from build123d import *

# Parameters (mm, degrees)
F1_DEPTH = 6.8
F3_DEPTH = 25
F5_DEPTH = 2
F7_DEPTH = 2


with BuildPart() as f1:
    # F0 (on Top) → F1 (new body)
    with BuildSketch(Plane.XY):
        with BuildLine():
            ThreePointArc((-46.538709, 10.046789), (-53.609776, 7.117857), (-56.538709, 0.046789))
            Line((-56.538709, 0.046789), (-37.538709, 0.046789))
            Line((-37.538709, 0.046789), (-37.538709, 10.046789))
            Line((-37.538709, 10.046789), (-46.538709, 10.046789))
        make_face()
        with BuildLine():
            Line((-37.538709, 0.046789), (-56.538709, 0.046789))
            ThreePointArc((-56.538709, 0.046789), (-53.609776, -7.024279), (-46.538709, -9.953211))
            Line((-46.538709, -9.953211), (-37.538709, -9.953211))
            Line((-37.538709, -9.953211), (-37.538709, 0.046789))
        make_face()
        with BuildLine():
            Line((-37.538709, 10.046789), (-37.538709, 0.046789))
            Line((-37.538709, 0.046789), (-18.538709, 0.046789))
            ThreePointArc((-18.538709, 0.046789), (-21.467641, 7.117857), (-28.538709, 10.046789))
            Line((-28.538709, 10.046789), (-37.538709, 10.046789))
        make_face()
        with BuildLine():
            Line((-18.538709, 0.046789), (-37.538709, 0.046789))
            Line((-37.538709, 0.046789), (-37.538709, -9.953211))
            Line((-37.538709, -9.953211), (-28.538709, -9.953211))
            ThreePointArc((-28.538709, -9.953211), (-21.467641, -7.024279), (-18.538709, 0.046789))
        make_face()
    extrude(amount=F1_DEPTH)

    # F2 (on face) → F3 (cut)
    with BuildSketch(Plane.XZ.offset(9.953211)):
        with BuildLine():
            Line((-46.538709, 6.8), (-46.538709, 4.885035))
            add(Edge.make_bspline(
                [(-46.538709, 4.885035), (-37.538709, 3.536233), (-28.538709, 4.885035)],
                knots=[4.014167, 4.014167, 4.014167, 5.410611, 5.410611, 5.410611], degree=2, weights=[1, 0.765986, 1]))
            Line((-28.538709, 4.885035), (-28.538709, 6.8))
            Line((-28.538709, 6.8), (-46.538709, 6.8))
        make_face()
        with BuildLine():
            add(Edge.make_bspline(
                [(-28.538709, 4.885035), (-23.538709, 5.634369), (-23.538709, 6.8)],
                knots=[5.410611, 5.410611, 5.410611, 6.283185, 6.283185, 6.283185], degree=2, weights=[1, 0.906327, 1]))
            add(Edge.make_bspline(
                [(-23.538709, 6.8), (-23.538709, 10.724017), (-43.454788, 9.065817), (-63.370868, 7.407617), (-46.538709, 4.885035)],
                knots=[0, 0, 0, 2.007083, 2.007083, 4.014167, 4.014167, 4.014167], degree=2, weights=[1, 0.537319, 1, 0.537319, 1]))
            Line((-46.538709, 4.885035), (-46.538709, 6.8))
            Line((-46.538709, 6.8), (-28.538709, 6.8))
            Line((-28.538709, 6.8), (-28.538709, 4.885035))
        make_face()
    extrude(amount=-F3_DEPTH, mode=Mode.SUBTRACT)

    # F4 (on face) → F5 (cut)
    with BuildSketch(Plane(origin=(0, 0, 0), x_dir=(1, 0, 0), z_dir=(0, 0, -1))):
        with BuildLine():
            Line((-28.538709, 9.353211), (-46.538709, 9.353211))
            ThreePointArc((-46.538709, 9.353211), (-55.938709, -0.046789), (-46.538709, -9.446789))
            Line((-46.538709, -9.446789), (-28.538709, -9.446789))
            ThreePointArc((-28.538709, -9.446789), (-19.138709, -0.046789), (-28.538709, 9.353211))
        make_face()
    extrude(amount=-F5_DEPTH, mode=Mode.SUBTRACT)

    # F6 (on face) → F7 (cut)
    with BuildSketch(Plane(origin=(0, 0, 2), x_dir=(1, 0, 0), z_dir=(0, 0, -1))):
        with BuildLine():
            Line((-28.538709, 3.953211), (-46.538709, 3.953211))
            ThreePointArc((-46.538709, 3.953211), (-50.538709, -0.046789), (-46.538709, -4.046789))
            Line((-46.538709, -4.046789), (-28.538709, -4.046789))
            ThreePointArc((-28.538709, -4.046789), (-24.538709, -0.046789), (-28.538709, 3.953211))
        make_face()
    extrude(amount=-F7_DEPTH, mode=Mode.SUBTRACT)


solid = f1.part
The listing builds one solid part. Answer for the finished solid, in the listing's coordinates (mm). A direction names the side the tool comes from. Give positions to 0.01 mm unless a question says otherwise; leave off trailing zeros. Loops run counter-clockwise (first coordinate to the right, second up) from the corner with the lowest first, then second, coordinate; pieces in that order, holes last.
Item 1: Each of these flat-tipped pins is pushed along its axis until it touches: pin 1 Ø5.5 at (x, y) = (-28.5, 0.5) entering from -Z; pin 2 Ø2 at (x, z) = (-51, 2.5) entering from +Y; pin 3 Ø3 at (x, z) = (-24.5, 2.5) entering from -Y. Where does it stop, or does it pass through?
Derived:
pin 1: stops at z = 4
pin 2: stops at y = 9.43
pin 3: stops at y = -9.63
Item 2: A cutting plane is placed at B-B (x = -22.5). Give the vertices of the cut face in (y, z).
Derived:
outline: (-7.92, 0) - (-7.16, 0) - (-7.16, 2) - (7.25, 2) - (7.25, 0) - (8.02, 0) - (8.02, 6.8) - (-7.92, 6.8) - close
Item 3: Find the intervals of material crossed by line 1 along Y through (x, z) = (-42, 1.75); line 2 along Y through (x, z) = (-28, 1.75); line 3 along X through (y, z) = (2.25, 6), in increasing order.
Derived:
line 1: y = -9.95 to -9.35, 9.45 to 10.05
line 2: y = -9.94 to -9.34, 9.43 to 10.03
line 3: x = -56.29 to -50.8, -24.27 to -18.78
Item 4: Determine the mould class of faces 1 (the cylindrical face through (-50.538, -0.041, 2.986)), 2 (the flat face through (-39, 9.7, 0)) for opening direction X: +X half, -X half, draft (parallel to the pull), parting line (faces both ways), or undercut.
Derived:
face 1: undercut
face 2: draft
Item 5: A cutting plane is placed at A-A (z = 1.5). Give the vertices of the cut face in (x, y), then the cut area to 3 significant figures.
Derived:
outline: (-56.54, 0.05) arc R10 ccw to (-46.54, -9.95) - (-28.54, -9.95) arc R10 ccw to (-18.54, 0.05) arc R10 ccw to (-28.54, 10.05) - (-46.54, 10.05) arc R10 ccw to start; hole (-46.54, -9.35) - (-28.54, -9.35) arc R9.4 ccw to (-28.54, 9.45) - (-46.54, 9.45) arc R9.4 ccw to start
area: 58.2 mm2
Item 6: A tool of negligible diameter and unlimited length cuts with its end or side. For faces 3 (the flat face through (-38, 0, 4)), 4 (the flat face through (-54, 0, 6.8)), from which of +Z, -Z, +X, -X, +Y, -Y can it reach the whole face along a straight path? Write none if from no direction.
Derived:
face 3: -Z
face 4: +Z, +X, -X, +Y, -Y
Item 7: A cutting plane is placed at C-C (x = -52). Give the vertices of the cut face in (y, z), then the cut area to 3 significant figures.
Derived:
outline: (-8.33, 0) - (-7.6, 0) - (-7.6, 2) - (7.7, 2) - (7.7, 0) - (8.42, 0) - (8.42, 6.8) - (-8.33, 6.8) - close
area: 83.3 mm2
